Verification items for the finished model (mm, model axes). A direction names the side the tool comes from. Give positions to 0.01 mm unless a question says otherwise; leave off trailing zeros. Loops run counter-clockwise (first coordinate to the right, second up) from the corner with the lowest first, then second, coordinate; pieces in that order, holes last. Notation, with made-up numbers: (23, 68) - (80, 68) arc R24 cw to (80, 88) - close; hole circle Ø6 at (59.5, -18). An arc over 180 degrees is marked (long way). Use one line per item in the form item = value.
```python
from build123d import *

# Parameters (mm, degrees)
F0_R      = 67.389458
F1_DEPTH  = 101.6
F2_R      = 12.788908
F3_DEPTH  = 161.798
F4_R      = 12.50156
F5_DEPTH  = 121.666
F6_R      = 5.08
F7_SIZE   = 5.08
F8_W      = 35.13822
F8_H      = 27.752711
F9_DEPTH  = 223.266
F10_W     = 102.441065
F10_H     = 36.250696
F11_DEPTH = 25.4
F12_DEPTH = 123.444


with BuildPart() as f1:
    # F0 (on Top) → F1 (new body)
    with BuildSketch(Plane.XY):
        with Locations((0, -3.060437)):
            Circle(F0_R)
    extrude(amount=F1_DEPTH)

    # F2 (on face) → F3 (cut)
    with BuildSketch(Plane.XY.offset(101.6)):
        Circle(F2_R)
    extrude(amount=-F3_DEPTH, mode=Mode.SUBTRACT)

    # F4 (on face) → F5 (cut)
    with BuildSketch(Plane.XY.offset(101.6)):
        with Locations((0, 45.001123)):
            Circle(F4_R)
    extrude(amount=-F5_DEPTH, mode=Mode.SUBTRACT)

    # F6
    f6_edges = [f1.edges().sort_by_distance(p)[0] for p in [
        (-67.389458, -3.060437, 101.6),
    ]]
    fillet(f6_edges, radius=F6_R)

    # F7
    f7_edges = [f1.edges().sort_by_distance(p)[0] for p in [
        (-67.389458, -3.060437, 0),
    ]]
    chamfer(f7_edges, length=F7_SIZE)

    # F8 (on face) → F9 (cut)
    with BuildSketch(Plane(origin=(0, 0, 0), x_dir=(1, 0, 0), z_dir=(0, 0, -1))):
        with Locations((2.640987, 35.737217)):
            Rectangle(F8_W, F8_H)
    extrude(amount=-F9_DEPTH, mode=Mode.SUBTRACT)

    # F10 (on Front) → F11 (join)
    with BuildSketch(Plane.XZ):
        with Locations((-16.654189, 58.523156)):
            Rectangle(F10_W, F10_H)
    extrude(amount=F11_DEPTH)

    # F10 (on Front) → F12 (join)
    with BuildSketch(Plane.XZ):
        with Locations((-16.654189, 58.523156)):
            Rectangle(F10_W, F10_H)
    extrude(amount=F12_DEPTH)


solid = f1.part
```
1. Scan lines: probe 1 along Y at (x, z) = (0, 56); probe 2 along Y at (x, z) = (0, 92.5); probe 3 along Y at (x, z) = (5, 74). Record each from-to range of solid material in increasing order.
Result set:
probe_1 = -123.44 to 0, 12.79 to 32.5, 57.5 to 64.33
probe_2 = -70.45 to -49.61, -21.86 to -12.79, 12.79 to 32.5, 57.5 to 64.33
probe_3 = -123.44 to 0, 11.77 to 33.54, 56.46 to 64.14
2. Section check A-A, the plane x = 0. State how many separate pieces and enclosed holes the cut face has, then the cut area to 3 significant figures.
Result set:
separate_pieces = 3
enclosed_holes = 0
area = 9,090 mm²
3. Depth check by flat-ended pin: pin 1 Ø10 at (x, y) = (4.5, -5.5) entering from +Z; pin 2 Ø14 at (x, y) = (2.5, -30.5) entering from -Z; pin 3 Ø1.5 at (y, z) = (-59.5, 80.5) entering from +X. Enter the tip coordinate at first touch or a pass-through.
Result set:
pin_1 = 76.65
pin_2 = 40.4
pin_3 = 37.95
4. Draft check along X on faces 6 (the flat face through (13, -2, 0)), 7 (the cylindrical face through (5.77, 33.91, 51.51)), 8 (the cylindrical face through (36.23, 53.76, 50.16)). Enter one of: released by +X, released by -X, zero draft, split by the parting line, or undercut.
Result set:
face_6 = zero draft
face_7 = undercut
face_8 = split by the parting line
5. Tool access check on faces 1 (the flat face through (20.21, -36, 20)), 2 (the flat face through (34.566, -92, 58)), 3 (the flat face through (2, -21.861, 89)), 4 (the flat face through (-17, -123.444, 59)), 5 (the flat face through (0, 0, 59)). Record the directions out of +Z, -Z, +X, -X, +Y, -Y that give a thin tool (end or side, any length) a straight path to the whole face; none if there is none.
Result set:
face_1 = -Z
face_2 = +Z, -Z, +X, -Y
face_3 = +Z
face_4 = +Z, -Z, +X, -X, -Y
face_5 = +Z, -Z
6. Section check C-C, the plane y = -85. Record the cut outline in (x, z).
Result set:
outline = (-67.87, 40.4) - (34.57, 40.4) - (34.57, 76.65) - (-67.87, 76.65) - close
7. Section check B-B, the plane z = 46.5. Record the cut outline in (x, y).
Result set:
outline = (-67.87, -123.44) - (34.57, -123.44) - (34.57, -60.91) arc R67.39 ccw (long way) to (-67.32, 0) - (-67.87, 0) - close; hole (-12.79, 0) - (12.79, 0) arc R12.79 ccw to start; hole circle Ø25 at (0, 45)
